from build123d import *

# Parameters (mm, degrees)
SKETCH_1_R      = 1
EXTRUDE_1_DEPTH = 0.5
EXTRUDE1_DEPTH  = 0.5
EXTRUDE2_DEPTH  = 0.5
FILLET8_R       = 1
FILLET9_R       = 1


with BuildPart() as part:
    # Эскиз1 → Бобышка-Вытянуть1 (new, symmetric)
    with BuildSketch(Plane.XY):
        with BuildLine():
            Line((0, 2), (-25.5979, 2))
            ThreePointArc((-25.5979, 2), (-27.5979, 0), (-25.5979, -2))
            Line((-25.5979, -2), (0, -2))
            ThreePointArc((0, -2), (2, 0), (0, 2))
        make_face()
        with Locations((-25.5979, 0)):
            Circle(SKETCH_1_R, mode=Mode.SUBTRACT)
        Circle(SKETCH_1_R, mode=Mode.SUBTRACT)
    extrude(amount=EXTRUDE_1_DEPTH, both=True)

    # Sketch1 → Extrude1 (add, symmetric)
    with BuildSketch(Plane.XY):
        Polygon((-8.843145751, 2), (-12.343145751, 5.5), (-15.656854249, 5.5), (-19.156854249, 2), align=None)
    extrude(amount=EXTRUDE1_DEPTH, both=True)

    # Sketch → Extrude2 (cut, symmetric)
    with BuildSketch(Plane.XY):
        Polygon((-10.5, -2), (-14, 1.5), (-17.5, -2), align=None)
    extrude(amount=EXTRUDE2_DEPTH, both=True, mode=Mode.SUBTRACT)

    # Fillet8
    fillet8_edges = [part.edges().sort_by_distance(p)[0] for p in [
        (-8.843145751, 2, 0),
        (-19.156854249, 2, 0),
        (-14, 1.5, 0),
    ]]
    fillet(fillet8_edges, radius=FILLET8_R)

    # Fillet9
    fillet9_edges = [part.edges().sort_by_distance(p)[0] for p in [
        (-15.656854249, 5.5, 0),
        (-12.343145751, 5.5, 0),
        (-17.5, -2, 0),
        (-10.5, -2, 0),
    ]]
    fillet(fillet9_edges, radius=FILLET9_R)


solid = part.part
The model under review builds one solid part; all positions refer to its coordinate system, in mm. A direction names the side the tool comes from. Round coordinates to 2 decimals unless told otherwise and drop trailing zeros. Write each loop counter-clockwise with the first axis right and the second up, starting at its lowest first coordinate (ties: lowest second). Pieces come first, ordered by that corner, then holes. Notation, with made-up numbers: (32.5, -1) - (60.5, -1) arc R26 cw to (60.5, 35) - close; hole circle Ø8 at (-9, 73). An arc over 180 degrees is marked (long way). One line per item, written item: value. Start each with the question number.
1. Clearance check with a flat-ended pin moving along its axis: P1, Ø1.6, axis at x = -25.6, y = 0, coming from the +Z side. State where the tip first meets the part, or that it passes through.
2. Consider section B-B on z = 0.05. Write out the cut boundary in (x, y), and give its area (3 significant figures).
3. Machinability: for faces 4 (the face through (-5, -2, 0)), 5 (the face through (-23, 2, 0)), 6 (the face through (-24.674, -0.383, -0.007)), 7 (the face through (-12, -0.5, 0)), 8 (the face through (-4, 2, 0)), which of the approach directions +Z, -Z, +X, -X, +Y, -Y give a long, thin tool a straight path to every point of the face, cutting with its end or side? Answer none if there is none.
4. Consider section A-A on y = 0. Write out the cut boundary in (x, z).
5. Consider section D-D on y = 4.5. Write out the cut boundary in (x, z).
6. The part is to be moulded in two halves that separate along X. For faces 1 (the face through (-15.9, -0.4, 0)), 2 (the face through (-14, 5.5, 0)), 3 (the face through (-10.573, 3.73, 0.007)), say which applies: released by +X, released by -X, zero draft, split by the parting line, or undercut.
7. To check wall thickness, follow L1, parallel to Y at x = -5, z = -0.4; L2, parallel to X at y = 0.75, z = -0.1; L3, parallel to Y at x = -15.5, z = -0.25. State the ranges of each line that lie inside material, in increasing order. Write a range as from..to.
8. Consider section C-C on x = -5.5. Write out the cut boundary in (y, z), and give its area (3 significant figures).
Checks:
1. P1: passes through
2. outline: (-25.6, -2) - (-17.91, -2) arc R1 ccw to (-17.21, -1.71) - (-14.71, 0.79) arc R1 cw to (-13.29, 0.79) - (-10.79, -1.71) arc R1 ccw to (-10.09, -2) - (0, -2) arc R2 ccw to (0, 2) - (-8.43, 2) arc R1 cw to (-9.14, 2.29) - (-12.05, 5.21) arc R1 ccw to (-12.76, 5.5) - (-15.24, 5.5) arc R1 ccw to (-15.95, 5.21) - (-18.86, 2.29) arc R1 cw to (-19.57, 2) - (-25.6, 2) arc R2 ccw to start; hole circle Ø2 at (-25.6, 0); hole circle Ø2 at (0, 0)
2. area: 120 mm^2
3. face 4: +Z, -Z, +X, -X, -Y
3. face 5: +Z, -Z, -X, +Y
3. face 6: +Z, -Z
3. face 7: +Z, -Z, -Y
3. face 8: +Z, -Z, +X, +Y
4. outline: (-27.6, -0.5) - (-26.6, -0.5) - (-26.6, 0.5) - (-27.6, 0.5) - close; (-24.6, -0.5) - (-15.5, -0.5) - (-15.5, 0.5) - (-24.6, 0.5) - close; (-12.5, -0.5) - (-1, -0.5) - (-1, 0.5) - (-12.5, 0.5) - close; (1, -0.5) - (2, -0.5) - (2, 0.5) - (1, 0.5) - close
5. outline: (-16.66, -0.5) - (-11.34, -0.5) - (-11.34, 0.5) - (-16.66, 0.5) - close
6. face 1: undercut
6. face 2: zero draft
6. face 3: released by +X
7. L1: y = -2..2
7. L2: x = -27.45..-26.26, -24.94..-14.75, -13.25..-0.66, 0.66..1.85
7. L3: y = 0..5.47
8. outline: (-2, -0.5) - (2, -0.5) - (2, 0.5) - (-2, 0.5) - close
8. area: 4.00 mm^2
